Geometry check sheet. Reference: drawing and pictorial views, mm from the part's lowest x, y, z. Round coordinates to 2 decimals unless told otherwise and drop trailing zeros. Write each loop counter-clockwise with the first axis right and the second up, starting at its lowest first coordinate (ties: lowest second). Pieces come first, ordered by that corner, then holes. Notation, with made-up numbers: M 87,47 L 126,47 A9 ccw 126,56 Z; hole C -20,77.5 d6. An arc over 180 degrees is marked long. Answer in a Markdown table with one row per item.
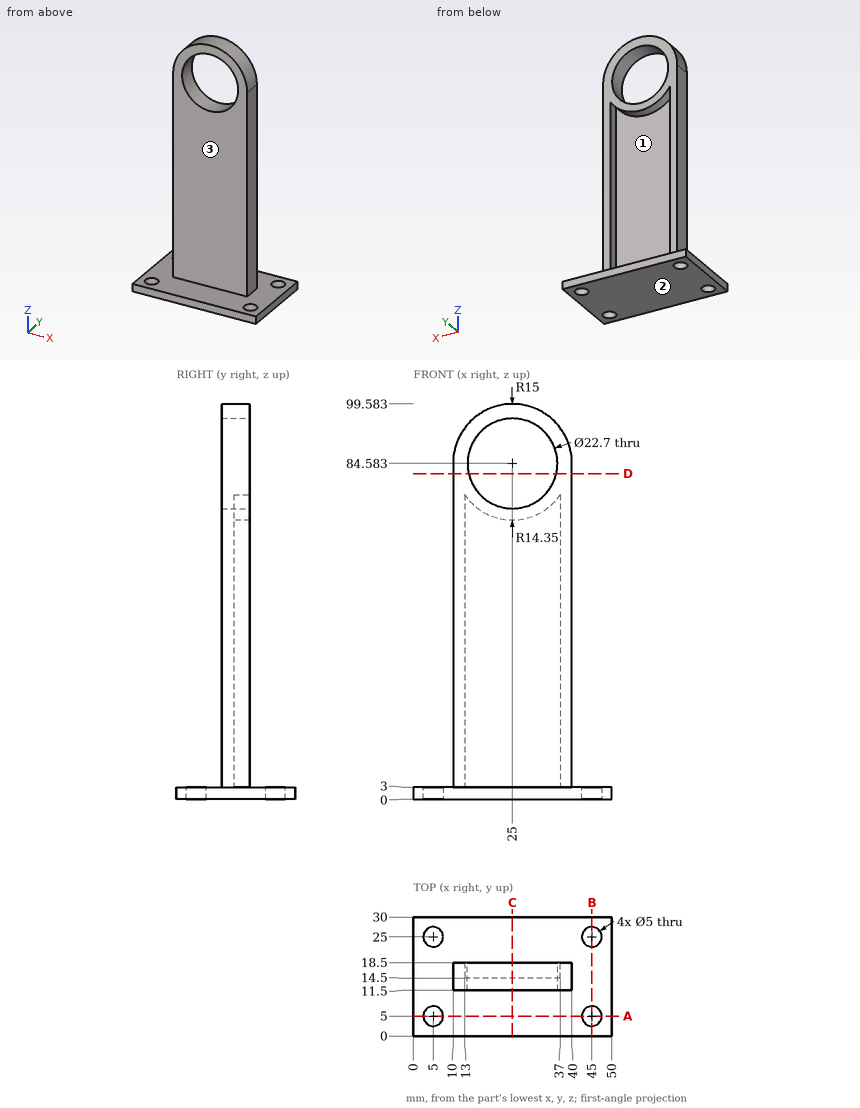
1. Go/stop test with flat-tipped pins: pin 1 (7.5 mm diameter, centred on y = 15.5, z = 56, fed in from +X); pin 2 (4 mm diameter, centred on x = 5, y = 5, fed in from -Z); pin 3 (12 mm diameter, centred on x = 12.5, y = 11, fed in from -Z); pin 4 (6 mm diameter, centred on x = 5, y = 25, fed in from +Z). Record where each tip stops, or that it passes through.
Found:
| item | result |
|---|---|
| pin 1 | stops at x = 40 |
| pin 2 | passes through |
| pin 3 | stops at z = 0 |
| pin 4 | stops at z = 3 |
2. Scan lines: L1, parallel to Y at x = 45, z = 2.4; L2, parallel to Y at x = 34, z = 94; L3, parallel to Z at x = 46.5, y = 12.75. Record each from-to range of solid material in increasing order.
Found:
| item | result |
|---|---|
| L1 | y = 0 to 2.5, 7.5 to 22.5, 27.5 to 30 |
| L2 | y = 11.5 to 18.5 |
| L3 | z = 0 to 3 |
3. Section check D-D, the plane z = 82. Record the cut outline in (x, y).
Found:
| item | result |
|---|---|
| outline | M 10,11.5 L 13.95,11.5 L 13.95,18.5 L 10,18.5 Z; M 36.05,11.5 L 40,11.5 L 40,18.5 L 36.05,18.5 Z |
4. Section check C-C, the plane x = 25. Record the cut outline in (y, z).
Found:
| item | result |
|---|---|
| outline | M 0,0 L 30,0 L 30,3 L 14.5,3 L 14.5,70.23 L 18.5,70.23 L 18.5,73.23 L 11.5,73.23 L 11.5,3 L 0,3 Z; M 11.5,95.93 L 18.5,95.93 L 18.5,99.58 L 11.5,99.58 Z |
5. Draft check along Z on the marked faces 1, 2 and 3. Enter one of: +Z half, -Z half, draft (parallel to the pull), parting line (faces both ways), or undercut.
Found:
| item | result |
|---|---|
| face 1 | undercut |
| face 2 | -Z half |
| face 3 | draft |
6. Section check A-A, the plane y = 5. Record the cut outline in (x, z).
Found:
| item | result |
|---|---|
| outline | M 0,0 L 2.5,0 L 2.5,3 L 0,3 Z; M 7.5,0 L 42.5,0 L 42.5,3 L 7.5,3 Z; M 47.5,0 L 50,0 L 50,3 L 47.5,3 Z |
7. Section check B-B, the plane x = 45. Record the cut outline in (y, z).
Found:
| item | result |
|---|---|
| outline | M 0,0 L 2.5,0 L 2.5,3 L 0,3 Z; M 7.5,0 L 22.5,0 L 22.5,3 L 7.5,3 Z; M 27.5,0 L 30,0 L 30,3 L 27.5,3 Z |
